The figure shows three views and two pictorial views of one solid part (mm, origin at its lowest corner). Answer the questions. Coordinates: 2 decimals unless noted, no trailing zeros. Order: outer loops, then holes, each group sorted by start corner. A loop starts at its lowest first (then second) coordinate and runs counter-clockwise, first axis right, second up. Notation, with made-up numbers: (-19.75, -4) -> (23.25, -4) arc R15 ccw to (23.25, 22) -> close; hole circle Ø8 at (-35, 31.25). An arc over 180 degrees is marked (long way). Return JSON: item names as keys, results as strings.
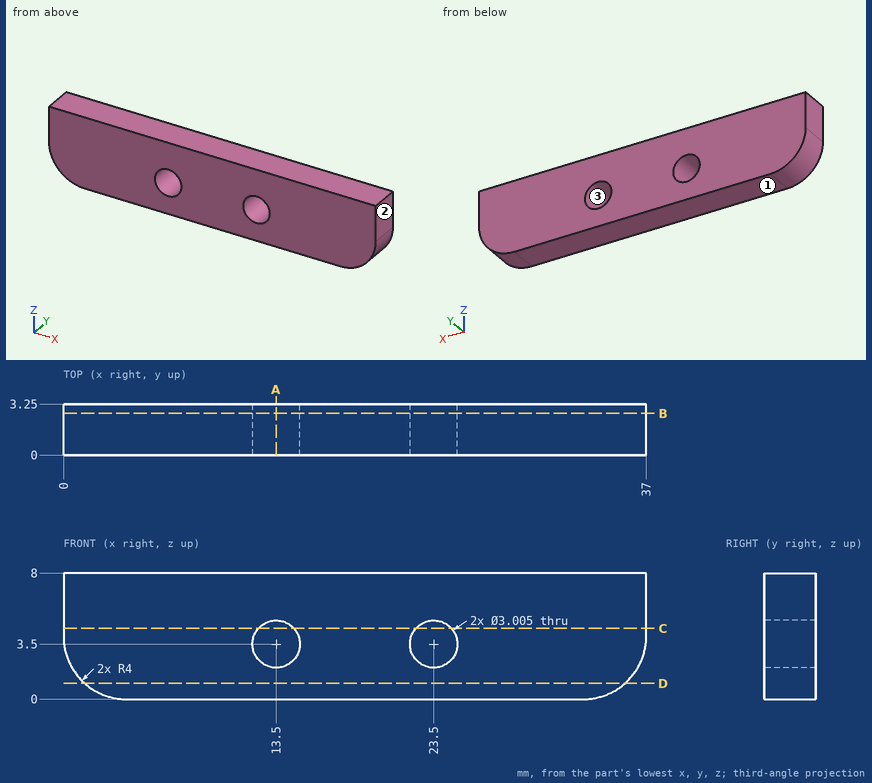
Item 1: Flat-ended cylindrical pins translate along their axes: pin 1 (2.5 mm diameter, centred on x = 23.5, z = 3.5, fed in from -Y); pin 2 (4 mm diameter, centred on x = 13.5, z = 4, fed in from +Y). Find the tip coordinate at first contact, or state that the pin passes through.
Answer list:
{"pin 1": "through", "pin 2": "y = 3.25"}
Item 2: Determine the mould class of the marked faces 1, 2 and 3 for opening direction X: pulls with the +X half, pulls with the -X half, needs draft (parallel to the pull), parting line crosses it, or undercut.
Answer list:
{"face 1": "needs draft", "face 2": "pulls with the +X half", "face 3": "undercut"}
Item 3: Find the intervals of material crossed by probe 1 along Z at (x, y) = (23.5, 1.65); probe 2 along X at (y, z) = (1.05, 3.5); probe 3 along X at (y, z) = (1.8, 3), in increasing order.
Answer list:
{"probe 1": "0 to 2, 5 to 8", "probe 2": "0.03 to 12, 15 to 22, 25 to 36.97", "probe 3": "0.13 to 12.08, 14.92 to 22.08, 24.92 to 36.87"}
Item 4: The part is cut by section D-D on z = 1. Determine the outline of the cut face in (x, y).
Answer list:
{"outline": "(1.35, 0) -> (35.65, 0) -> (35.65, 3.25) -> (1.35, 3.25) -> close"}
Item 5: The part is cut by section A-A on x = 13.5. Determine the outline of the cut face in (y, z).
Answer list:
{"outline": "(0, 0) -> (3.25, 0) -> (3.25, 2) -> (0, 2) -> close; (0, 5) -> (3.25, 5) -> (3.25, 8) -> (0, 8) -> close"}
Item 6: The part is cut by section C-C on z = 4.5. Determine the outline of the cut face in (x, y).
Answer list:
{"outline": "(0, 0) -> (12.38, 0) -> (12.38, 3.25) -> (0, 3.25) -> close; (14.62, 0) -> (22.38, 0) -> (22.38, 3.25) -> (14.62, 3.25) -> close; (24.62, 0) -> (37, 0) -> (37, 3.25) -> (24.62, 3.25) -> close"}
Item 7: The part is cut by section B-B on y = 2.65. Determine the outline of the cut face in (x, z) (1 decimal), plus the area to 3 significant figures.
Answer list:
{"outline": "(0, 4) arc R4 ccw to (4, 0) -> (33, 0) arc R4 ccw to (37, 4) -> (37, 8) -> (0, 8) -> close; hole circle Ø3 at (13.5, 3.5); hole circle Ø3 at (23.5, 3.5)", "area": "275 mm2"}
